Geometry: final body of the model. Coordinates: model frame, mm. A direction names the side the tool comes from. Round coordinates to 2 decimals unless told otherwise and drop trailing zeros. Write each loop counter-clockwise with the first axis right and the second up, starting at its lowest first coordinate (ties: lowest second). Pieces come first, ordered by that corner, then holes. Notation, with made-up numbers: M 50,51.25 L 102,51.25 A22 cw 102,76.25 Z; hole C 89,59 d3. An arc over 180 degrees is marked long. Put each result on its own line as item: value. Start each with the question number.
```python
from build123d import *

# Parameters (mm, degrees)
SKETCH1_R                = 11.5
SKETCH1_R_2              = 1.75
BOSS_EXTRUDE2_DEPTH      = 6
SKETCH2_W                = 4
SKETCH2_H                = 2
BOSS_EXTRUDE3_DEPTH      = 12
SKETCH3_R                = 35
SKETCH3_R_2              = 9
BOSS_EXTRUDE5_DEPTH      = 12
BOSS_EXTRUDE5_DEPTH_BACK = 1


with BuildPart() as part:
    # Sketch1 → Boss-Extrude2 (new body)
    with BuildSketch(Plane.XY):
        Circle(SKETCH1_R)
        with Locations((0, 6.5)):
            Circle(SKETCH1_R_2, mode=Mode.SUBTRACT)
        with Locations((6.5, 0)):
            Circle(SKETCH1_R_2, mode=Mode.SUBTRACT)
        with Locations((0, -6.5)):
            Circle(SKETCH1_R_2, mode=Mode.SUBTRACT)
        with Locations((-6.5, 0)):
            Circle(SKETCH1_R_2, mode=Mode.SUBTRACT)
    extrude(amount=BOSS_EXTRUDE2_DEPTH)

    # Sketch2 → Boss-Extrude3 (add)
    with BuildSketch(Plane.XY.offset(6)):
        with Locations((0, 10.324751653)):
            Rectangle(SKETCH2_W, SKETCH2_H)
        with BuildLine():
            Line((-2, 11.324751653), (2, 11.324751653))
            ThreePointArc((2, 11.324751653), (0, 11.5), (-2, 11.324751653))
        make_face()
        with BuildLine():
            ThreePointArc((8.807522623, -7.394426634), (9.959292144, -5.75), (10.807522623, -3.930325019))
            Line((10.807522623, -3.930325019), (8.807522623, -7.394426634))
        make_face()
        Polygon((8.807522623, -7.394426634), (7.075471815, -6.394426634), (9.075471815, -2.930325019), (10.807522623, -3.930325019), align=None)
        with BuildLine():
            ThreePointArc((-10.807522623, -3.930325019), (-9.959292144, -5.75), (-8.807522623, -7.394426634))
            Line((-8.807522623, -7.394426634), (-10.807522623, -3.930325019))
        make_face()
        Polygon((-10.807522623, -3.930325019), (-9.075471815, -2.930325019), (-7.075471815, -6.394426634), (-8.807522623, -7.394426634), align=None)
    extrude(amount=BOSS_EXTRUDE3_DEPTH)

    # Sketch3 → Boss-Extrude5 (add, two sides)
    with BuildSketch(Plane.XY.offset(18)) as boss_extrude5_sk:
        Circle(SKETCH3_R)
        with BuildLine():
            Line((-1.55765655, 27.455850125), (-1.55765655, 14.918904319))
            ThreePointArc((-1.55765655, 14.918904319), (-6.508256087, 13.514533019), (-10.692886106, 10.519609628))
            Line((-10.692886106, 10.519609628), (-20.494665031, 18.336267484))
            ThreePointArc((-20.494665031, 18.336267484), (-11.931802826, 24.776643867), (-1.55765655, 27.455850125))
        make_face(mode=Mode.SUBTRACT)
        with BuildLine():
            Line((-22.437030979, 15.900617624), (-12.635252054, 8.083959768))
            ThreePointArc((-12.635252054, 8.083959768), (-14.623918683, 3.337814009), (-14.89146743, -1.801165674))
            Line((-14.89146743, -1.801165674), (-27.11408583, -4.590898564))
            ThreePointArc((-27.11408583, -4.590898564), (-26.810517585, 6.119325684), (-22.437030979, 15.900617624))
        make_face(mode=Mode.SUBTRACT)
        with BuildLine():
            Line((-26.420863449, -7.628104261), (-14.198245049, -4.838371371))
            ThreePointArc((-14.198245049, -4.838371371), (-11.727472237, -9.352347028), (-7.876470048, -12.765626486))
            Line((-7.876470048, -12.765626486), (-13.316046972, -24.061024356))
            ThreePointArc((-13.316046972, -24.061024356), (-21.500365768, -17.145969551), (-26.420863449, -7.628104261))
        make_face(mode=Mode.SUBTRACT)
        with BuildLine():
            Line((-10.509246854, -25.412708052), (-5.069669931, -14.117310183))
            ThreePointArc((-5.069669931, -14.117310183), (0, -15), (5.069669931, -14.117310183))
            Line((5.069669931, -14.117310183), (10.509246854, -25.412708052))
            ThreePointArc((10.509246854, -25.412708052), (0, -27.5), (-10.509246854, -25.412708052))
        make_face(mode=Mode.SUBTRACT)
        with BuildLine():
            Line((13.316046972, -24.061024356), (7.876470048, -12.765626486))
            ThreePointArc((7.876470048, -12.765626486), (11.727472237, -9.352347028), (14.198245049, -4.838371371))
            Line((14.198245049, -4.838371371), (26.420863449, -7.628104261))
            ThreePointArc((26.420863449, -7.628104261), (21.500365768, -17.145969551), (13.316046972, -24.061024356))
        make_face(mode=Mode.SUBTRACT)
        with BuildLine():
            Line((27.11408583, -4.590898564), (14.89146743, -1.801165674))
            ThreePointArc((14.89146743, -1.801165674), (14.623918683, 3.337814009), (12.635252054, 8.083959768))
            Line((12.635252054, 8.083959768), (22.437030979, 15.900617624))
            ThreePointArc((22.437030979, 15.900617624), (26.810517585, 6.119325684), (27.11408583, -4.590898564))
        make_face(mode=Mode.SUBTRACT)
        with BuildLine():
            Line((20.494665031, 18.336267484), (10.692886106, 10.519609628))
            ThreePointArc((10.692886106, 10.519609628), (6.508256087, 13.514533019), (1.55765655, 14.918904319))
            Line((1.55765655, 14.918904319), (1.55765655, 27.455850125))
            ThreePointArc((1.55765655, 27.455850125), (11.931802826, 24.776643867), (20.494665031, 18.336267484))
        make_face(mode=Mode.SUBTRACT)
        Circle(SKETCH3_R_2, mode=Mode.SUBTRACT)
    extrude(amount=BOSS_EXTRUDE5_DEPTH)
    extrude(boss_extrude5_sk.sketch, amount=-BOSS_EXTRUDE5_DEPTH_BACK)


solid = part.part
```
1) Section B-B, the plane z = 7.5. Output: boundary loops of the cut face in (x, y).
2) Section D-D, the plane y = 6.5. Output: boundary loops of the cut face in (x, z).
3) Section A-A, the plane z = 24.5. Give the number of separate pieces and of enclosed holes in the cut face, and give its area (3 significant figures).
4) Access query for faces 5 (the face through (-1.172, 8.923, 23.409)), 6 (the face through (0, 0, 0)), 7 (the face through (0, 9.325, 11)), 8 (the face through (-2, 10, 11)), 9 (the face through (7.751, -19.686, 23.591)). Directions: +Z, -Z, +X, -X, +Y, -Y. A direction counts if a zero-diameter tool reaches every point of the face in a straight line with its end or side. Return the directions, or none.
5) First-contact query: pin 1 (4.5 mm diameter, centred on x = -0.5, z = 11, fed in from -Y); pin 2 (4 mm diameter, centred on y = 20.5, z = 26.5, fed in from -X); pin 3 (4.5 mm diameter, centred on x = 0, y = 6.5, fed in from +Z). Flat tips, straight axial feed; report the tip coordinate or a pass-through.
6) Section C-C, the plane x = 0. Output: boundary loops of the cut face in (y, z).
7) Ray query, probe 1 along Y at (x, z) = (0, 3.1); probe 2 along X at (y, z) = (1, 17.25); probe 3 along X at (y, z) = (17.5, 22.25). Return the intervals inside material, ascending.
8) Draft query along Y for faces 1 (the face through (7, -7, 17)), 2 (the face through (-0.38, 4.79, 2.96)), 3 (the face through (20.224, -6.214, 23.591)), 4 (the face through (-7.93, -6.89, 11.42)). Return one class per face: +Y half, -Y half, draft (parallel to the pull), parting line (faces both ways), or undercut.
Solved:
1. outline: M -10.81,-3.93 A11.5 ccw -8.81,-7.39 L -7.08,-6.39 L -9.08,-2.93 Z; M -2,9.32 L 2,9.32 L 2,11.32 A11.5 ccw -2,11.32 Z; M 7.08,-6.39 L 8.81,-7.39 A11.5 ccw 10.81,-3.93 L 9.08,-2.93 Z
2. outline: M -34.39,17 L -26.72,17 L -26.72,30 L -34.39,30 Z; M -13.52,17 L -6.22,17 L -6.22,30 L -13.52,30 Z; M -9.49,0 L -1.75,0 L -1.75,6 L -9.49,6 Z; M 1.75,0 L 9.49,0 L 9.49,6 L 1.75,6 Z; M 6.22,17 L 13.52,17 L 13.52,30 L 6.22,30 Z; M 26.72,17 L 34.39,17 L 34.39,30 L 26.72,30 Z
3. separate pieces: 1
3. enclosed holes: 8
3. area: 2,200 mm2
4. face 5: +Z
4. face 6: -Z, +X, -X, +Y, -Y
4. face 7: +X, -X, -Y
4. face 8: -X, +Y, -Y
4. face 9: +Z, -Z
5. pin 1: stops at y = 9.32
5. pin 2: stops at x = -29.71
5. pin 3: stops at z = 6
6. outline: M -35,17 L -27.5,17 L -27.5,30 L -35,30 Z; M -15,17 L -9,17 L -9,30 L -15,30 Z; M -11.5,0 L -8.25,0 L -8.25,6 L -11.5,6 Z; M -4.75,0 L 4.75,0 L 4.75,6 L -4.75,6 Z; M 8.25,0 L 11.5,0 L 11.5,17 L 35,17 L 35,30 L 9,30 L 9,17 L 9.32,17 L 9.32,6 L 8.25,6 Z
7. probe 1: y = -11.5 to -8.25, -4.75 to 4.75, 8.25 to 11.5
7. probe 2: x = -34.99 to -27.48, -14.97 to -8.94, 8.94 to 14.97, 27.48 to 34.99
7. probe 3: x = -30.31 to -19.45, -1.56 to 1.56, 19.45 to 30.31
8. face 1: draft
8. face 2: undercut
8. face 3: undercut
8. face 4: -Y half
